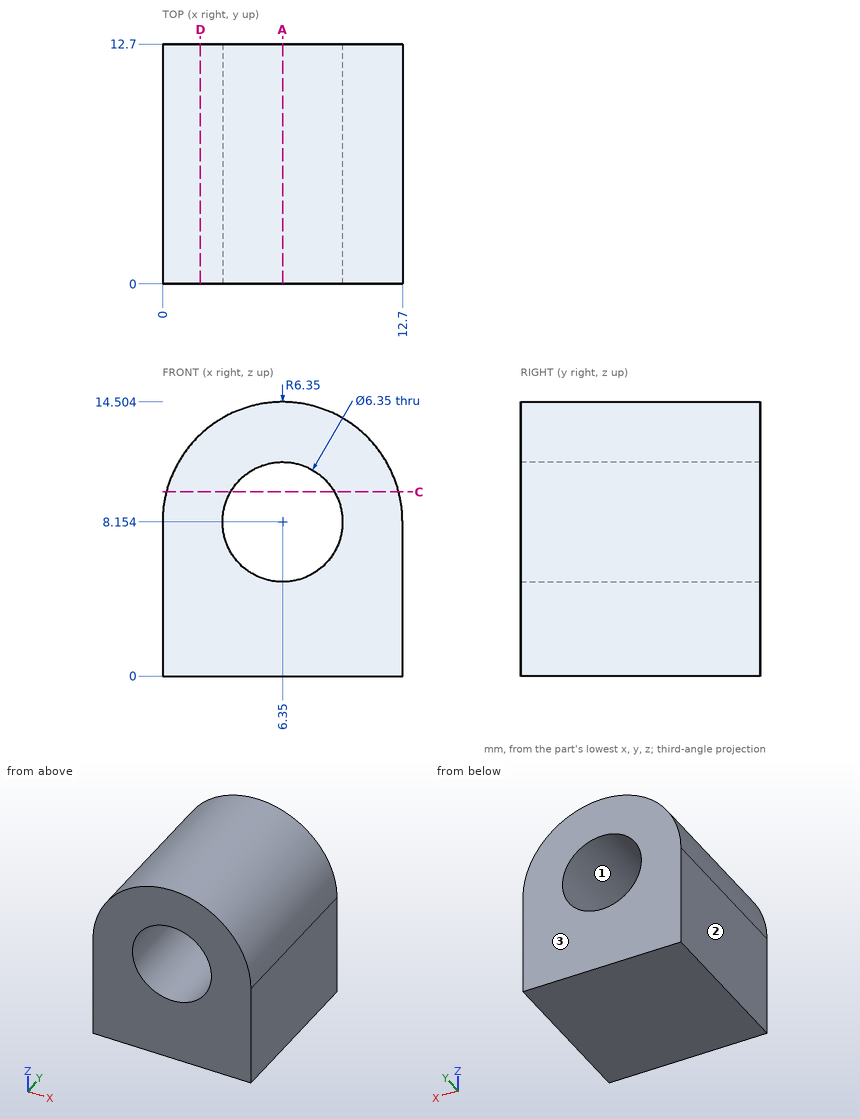
Part print with two shaded views. Sizes in mm from the minimum x, y, z corner. Coordinates: 2 decimals unless noted, no trailing zeros. Write each loop counter-clockwise with the first axis right and the second up, starting at its lowest first coordinate (ties: lowest second). Pieces come first, ordered by that corner, then holes. Notation, with made-up numbers: (-17.75, -3.75) - (-0.75, -3.75) arc R27 cw to (-0.75, 28.25) - close; hole circle Ø6 at (31, 85.25). An arc over 180 degrees is marked (long way). One line per item, written item: value. Start each with the question number.
1. Probe line 1 (Z direction, x = 6.5, y = 2) (1 decimal); line 2 (X direction, y = 4.5, z = 8); line 3 (X direction, y = 5.25, z = 5.75) (1 decimal). List the from-to ranges inside material, lowest first. Write a range as from..to.
2. Slice it at A-A (x = 6.35). Write the cut outline in (y, z).
3. Mould opens along X. For the marked faces 1, 2 and 3 say: released by +X, released by -X, zero draft, split by the parting line, or undercut.
4. Slice it at C-C (z = 9.75). Write the cut outline in (x, y) (1 decimal), plus the area to 3 significant figures.
5. Flat gauge pins, fed straight in: pin 1 (5 mm diameter, centred on y = 2.5, z = 11, fed in from +X); pin 2 (2 mm diameter, centred on y = 9.5, z = 11.5, fed in from +X). Where does each tip first touch, or does it go through?
6. Slice it at D-D (x = 2). Write the cut outline in (y, z).
Answers below:
1. line 1: z = 0..5, 11.3..14.5
1. line 2: x = 0..3.18, 9.52..12.7
1. line 3: x = 0..4.3, 8.4..12.7
2. outline: (0, 0) - (12.7, 0) - (12.7, 4.98) - (0, 4.98) - close; (0, 11.33) - (12.7, 11.33) - (12.7, 14.5) - (0, 14.5) - close
3. face 1: undercut
3. face 2: released by -X
3. face 3: zero draft
4. outline: (0.2, 0) - (3.6, 0) - (3.6, 12.7) - (0.2, 12.7) - close; (9.1, 0) - (12.5, 0) - (12.5, 12.7) - (9.1, 12.7) - close
4. area: 86.4 mm^2
5. pin 1: stops at x = 12.69
5. pin 2: stops at x = 12.25
6. outline: (0, 0) - (12.7, 0) - (12.7, 12.78) - (0, 12.78) - close
